Model file for the job. Use its own axes, mm. A direction names the side the tool comes from. Round coordinates to 2 decimals unless told otherwise and drop trailing zeros. Loops run counter-clockwise (first coordinate to the right, second up) from the corner with the lowest first, then second, coordinate; pieces in that order, holes last. Notation, with made-up numbers: (-23, -36) -> (23, -36) arc R13 cw to (23, -22) -> close; hole circle Ø5 at (-8, 46). An arc over 180 degrees is marked (long way). Use a Markdown table: item, result.
from build123d import *

# Parameters (mm, degrees)
EXTRUDE_1_DEPTH      = 26.5
EXTRUDE_1_DEPTH_BACK = 26.5
CUT_EXTRUDE_1_DEPTH  = 2.3
CUT_EXTRUDE_2_DEPTH  = 2.3
SKETCH_4_R           = 18.5
CUT_EXTRUDE_3_DEPTH  = 2.3
SKETCH_5_W           = 142.237580419
SKETCH_5_H           = 102.661015156
CUT_EXTRUDE_4_DEPTH  = 3.3


with BuildPart() as part:
    # Sketch 1 → Extrude 1 (new, two sides: drawn at the far end of the back side and taken through both)
    with BuildSketch(Plane.XY.offset(-EXTRUDE_1_DEPTH_BACK)):
        with BuildLine():
            Line((-26.5, 0), (32.24, 0))
            ThreePointArc((32.24, 0), (34.191614716, 0.808385284), (35, 2.76))
            Line((35, 2.76), (35, 17))
            Line((35, 17), (32.7, 17))
            Line((32.7, 17), (32.7, 4.6))
            ThreePointArc((32.7, 4.6), (32.026345597, 2.973654403), (30.4, 2.3))
            Line((30.4, 2.3), (-26.5, 2.3))
            Line((-26.5, 2.3), (-26.5, 0))
        make_face()
    extrude(amount=EXTRUDE_1_DEPTH + EXTRUDE_1_DEPTH_BACK)

    # Sketch 2 → Cut-Extrude 1 (cut)
    with BuildSketch(Plane(origin=(35, 0, 0), x_dir=(0, 0, -1), z_dir=(1, 0, 0))):
        with BuildLine():
            Line((-16.75, 6.75), (-15.25, 6.75))
            ThreePointArc((-15.25, 6.75), (-12.951902961, 7.701902961), (-12, 10))
            ThreePointArc((-12, 10), (-12.951902961, 12.298097039), (-15.25, 13.25))
            Line((-15.25, 13.25), (-16.75, 13.25))
            ThreePointArc((-16.75, 13.25), (-19.048097039, 12.298097039), (-20, 10))
            ThreePointArc((-20, 10), (-19.048097039, 7.701902961), (-16.75, 6.75))
        make_face()
    extrude(amount=-CUT_EXTRUDE_1_DEPTH, mode=Mode.SUBTRACT)

    # Sketch 3 → Cut-Extrude 2 (cut)
    with BuildSketch(Plane(origin=(35, 0, 0), x_dir=(0, 0, -1), z_dir=(1, 0, 0))):
        with BuildLine():
            Line((15.25, 6.75), (16.75, 6.75))
            ThreePointArc((16.75, 6.75), (19.048097039, 7.701902961), (20, 10))
            ThreePointArc((20, 10), (19.048097039, 12.298097039), (16.75, 13.25))
            Line((16.75, 13.25), (15.25, 13.25))
            ThreePointArc((15.25, 13.25), (12.951902961, 12.298097039), (12, 10))
            ThreePointArc((12, 10), (12.951902961, 7.701902961), (15.25, 6.75))
        make_face()
    extrude(amount=-CUT_EXTRUDE_2_DEPTH, mode=Mode.SUBTRACT)

    # Sketch 4 → Cut-Extrude 3 (cut)
    with BuildSketch(Plane(origin=(0, 0, 0), x_dir=(1, 0, 0), z_dir=(0, 1, 0))):
        with Locations(Location((0, 0, 0), (0, 0, 270))):
            Circle(SKETCH_4_R)
    extrude(amount=CUT_EXTRUDE_3_DEPTH, mode=Mode.SUBTRACT)

    # Sketch 5 → Cut-Extrude 4 (cut)
    with BuildSketch(Plane(origin=(35, 0, 0), x_dir=(0, 0, -1), z_dir=(1, 0, 0))):
        with Locations((4.017170159, 13.868386078)):
            Rectangle(SKETCH_5_W, SKETCH_5_H)
        with BuildLine():
            Line((-26.5, 0), (26.5, 0))
            Line((26.5, 0), (26.5, 13.6))
            ThreePointArc((26.5, 13.6), (25.504163056, 16.004163056), (23.1, 17))
            Line((23.1, 17), (-23.1, 17))
            ThreePointArc((-23.1, 17), (-25.504163056, 16.004163056), (-26.5, 13.6))
            Line((-26.5, 13.6), (-26.5, 0))
        make_face(mode=Mode.SUBTRACT)
    extrude(amount=-CUT_EXTRUDE_4_DEPTH, mode=Mode.SUBTRACT)


solid = part.part
Q1. Flat gauge pins, fed straight in: pin 1 (10 mm diameter, centred on x = -20, z = 2.5, fed in from +Y); pin 2 (3 mm diameter, centred on x = -20, y = 4.5, fed in from +Z); pin 3 (1.6 mm diameter, centred on x = 34, z = -16, fed in from -Y); pin 4 (3 mm diameter, centred on y = 12.5, z = -6.5, fed in from -X). Where does each tip first touch, or does it go through?
Results list:
| item | result |
|---|---|
| pin 1 | stops at y = 2.3 |
| pin 2 | passes through |
| pin 3 | stops at y = 0.17 |
| pin 4 | stops at x = 32.7 |
Q2. Band-saw the part on A-A, the plane z = 0. Give the cut face in (x, y).
Results list:
| item | result |
|---|---|
| outline | (-26.5, 0) -> (-18.5, 0) -> (-18.5, 2.3) -> (-26.5, 2.3) -> close; (18.5, 0) -> (32.24, 0) arc R2.76 ccw to (35, 2.76) -> (35, 17) -> (32.7, 17) -> (32.7, 4.6) arc R2.3 cw to (30.4, 2.3) -> (18.5, 2.3) -> close |
Q3. Tool access for faces 1 (the face through (34, 13.25, -16)), 2 (the face through (32.7, 11, 0)), 3 (the face through (-7.086, 1.134, 17.089)): list every direction of +Z, -Z, +X, -X, +Y, -Y with a clear straight run to the whole face (end or side of a thin tool).
Results list:
| item | result |
|---|---|
| face 1 | +X, -X |
| face 2 | +Z, -Z, -X, +Y |
| face 3 | +Y, -Y |
Q4. Pull direction Z, two halves, no side cores. Call faces 4 (the face through (34, 6.75, 16)), 5 (the face through (9, 2, 26.5)), 6 (the face through (15, 2.3, 11.4)), 7 (the face through (34, 13.25, 16)): released by +Z, released by -Z, zero draft, split by the parting line, or undercut.
Results list:
| item | result |
|---|---|
| face 4 | undercut |
| face 5 | released by +Z |
| face 6 | zero draft |
| face 7 | undercut |
Q5. Drill centre lines: L1, parallel to Y at x = 29, z = 24.5; L2, parallel to X at y = 11.75, z = 21.5; L3, parallel to X at y = 1.65, z = 0. Where is each one in solid material? Low to high. Write a range as from..to.
Results list:
| item | result |
|---|---|
| L1 | y = 0..2.3 |
| L2 | x = 32.7..35 |
| L3 | x = -26.5..-18.5, 18.5..34.77 |
Q6. Band-saw the part on D-D, the plane y = 9. Give the cut face in (x, z).
Results list:
| item | result |
|---|---|
| outline | (32.7, -26.5) -> (35, -26.5) -> (35, -19.84) -> (32.7, -19.84) -> close; (32.7, -12.16) -> (35, -12.16) -> (35, 12.16) -> (32.7, 12.16) -> close; (32.7, 19.84) -> (35, 19.84) -> (35, 26.5) -> (32.7, 26.5) -> close |
Q7. Band-saw the part on B-B, the plane x = 0. Give the cut face in (y, z).
Results list:
| item | result |
|---|---|
| outline | (0, -26.5) -> (2.3, -26.5) -> (2.3, -18.5) -> (0, -18.5) -> close; (0, 18.5) -> (2.3, 18.5) -> (2.3, 26.5) -> (0, 26.5) -> close |
Q8. Band-saw the part on C-C, the plane z = -22. Give the cut face in (x, y), plus the area to 3 significant figures.
Results list:
| item | result |
|---|---|
| outline | (-26.5, 0) -> (32.24, 0) arc R2.76 ccw to (35, 2.76) -> (35, 17) -> (32.7, 17) -> (32.7, 4.6) arc R2.3 cw to (30.4, 2.3) -> (-26.5, 2.3) -> close |
| area | 175 mm² |
